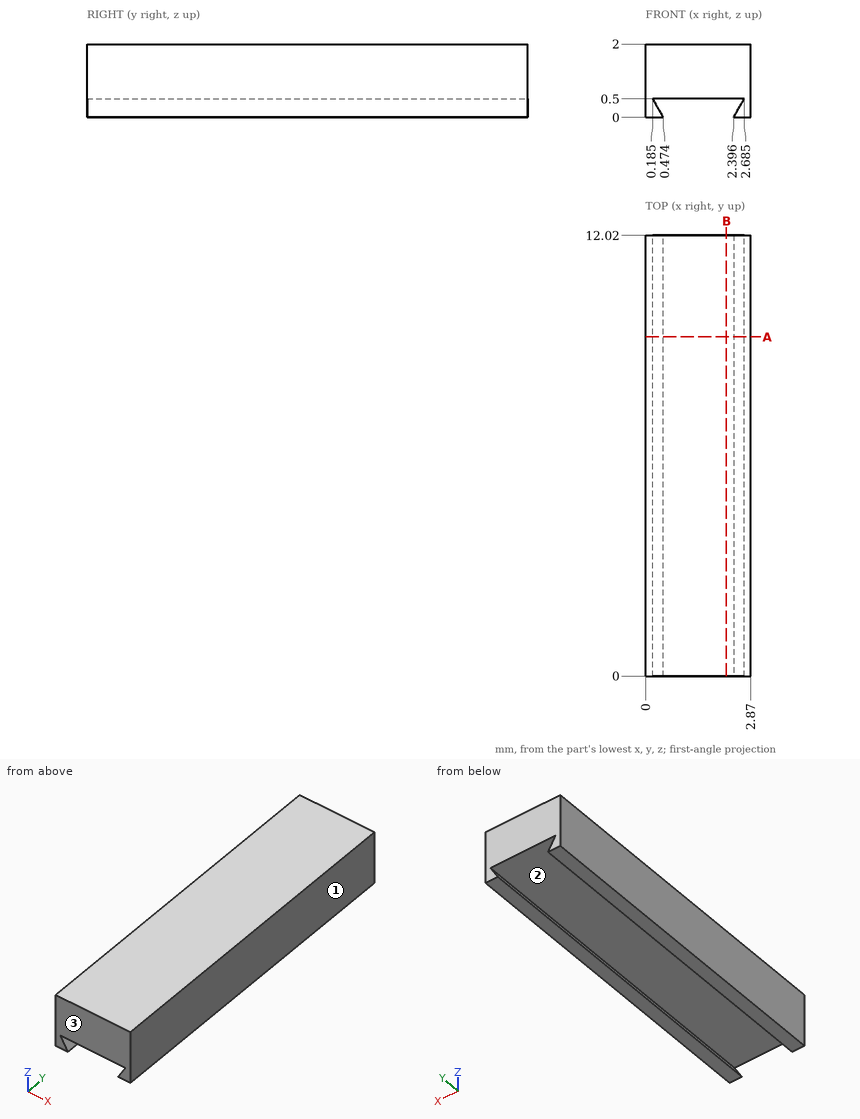
Geometry check sheet. Reference: drawing and pictorial views, mm from the part's lowest x, y, z. Round coordinates to 2 decimals unless told otherwise and drop trailing zeros. Order: outer loops, then holes, each group sorted by start corner. A loop starts at its lowest first (then second) coordinate and runs counter-clockwise, first axis right, second up. Notation, with made-up numbers: (1.25, 87.25) - (22.25, 87.25) arc R19 cw to (22.25, 117.25) - close; hole circle Ø11 at (65, 58.5). An arc over 180 degrees is marked (long way). One line per question, with ' | ' between items. Start each with the question number.
(1) Sectioned sample at B-B on x = 2.2. Record the cut outline in (y, z), and give its area (3 significant figures).
(2) Release check for a two-part mould opening along X. For the marked faces 1, 2 and 3 record: released by +X, released by -X, zero draft, split by the parting line, or undercut.
(3) Sectioned sample at A-A on y = 9.25. Record the cut outline in (x, z) (1 decimal).
(4) Thickness scan on L1, parallel to Z at x = 1.8, y = 9; L2, parallel to X at y = 7, z = 0.15. Record the ranges inside material, lowest first. Write a range as [from, to].
Conclusion:
1) outline: (0, 0.5) - (12.02, 0.5) - (12.02, 2) - (0, 2) - close | area: 18.0 mm2
2) face 1: released by +X | face 2: undercut | face 3: zero draft
3) outline: (0, 0) - (0.5, 0) - (0.2, 0.5) - (2.7, 0.5) - (2.4, 0) - (2.9, 0) - (2.9, 2) - (0, 2) - close
4) L1: z = [0.5, 2] | L2: x = [0, 0.39], [2.48, 2.87]
